Here's how the part is built. I have some questions about the finished solid (model axes, mm). A direction names the side the tool comes from. Give positions to 0.01 mm unless a question says otherwise; leave off trailing zeros. Loops run counter-clockwise (first coordinate to the right, second up) from the corner with the lowest first, then second, coordinate; pieces in that order, holes last. Notation, with made-up numbers: (42.25, -8.75) - (92.25, -8.75) arc R24 ccw to (92.25, 5.25) - close; hole circle Ø2 at (68.5, 71.25). An arc over 180 degrees is marked (long way). Return JSON: item names as keys, results as strings. Group by question number.
(1) For P1, Ø1, axis at y = -360.5, z = 8.5, coming from the -X side; P2, Ø6, axis at y = -316.5, z = 12, coming from the -X side; P3, Ø1.9, axis at y = -411, z = -2, coming from the -X side; P4, Ø8, axis at x = -9, y = -186, coming from the -Z side, each with a flat end and sliding along its axis, tell me the tip position at first contact or that it passes through.
(2) I need wall thicknesses on probe 1 along Y at (x, z) = (-5, 15); probe 2 along Y at (x, z) = (-1.5, 5.75); probe 3 along Z at (x, y) = (0, 1.25). Which ranges of each line are inside material? Lowest first, please. Write a range as [from, to].
(3) If we mould it in two halves opening along Y, with no side actions, what happens to faces 4 (the flat face through (0, -425.018, 6)), 5 (the cylindrical face through (0.385, -300.5, 16.688)), 6 (the flat face through (0, -205.181, 16))? For each: released by +Y, released by -Y, zero draft, split by the parting line, or undercut.
(4) If we section it at B-B (x = -3.5): Please give me the cut outline in (y, z), then the cut area to 3 significant figures.
(5) On a 3-axis mill with a long thin cutter (end or side, diameter ignored), from which of +Z, -Z, +X, -X, +Y, -Y can I reach the whole of each face in a straight line? I mean faces 1 (the cylindrical face through (-0.185, -335.118, 4.438)), 2 (the flat face through (-3, -398.526, 16)), 3 (the cylindrical face through (-0.23, -136.926, 6.495)). Say none if no direction works.
```python
from build123d import *
from build123d import SkipClean  # not in build123d's __all__

# Parameters (mm, degrees)
F1_DEPTH  = 29.21
F3_DEPTH  = 160.5534
F5_DEPTH  = 15.4178
F7_DEPTH  = 42.5196
F9_DEPTH  = 177.3174
F11_DEPTH = 26.4922
F13_DEPTH = 3.1496


with BuildPart() as f1:
    # F0 (on Front) → F1 (new body)
    with BuildSketch(Plane.XZ):
        with BuildLine():
            Line((11.9332703397, -4.6441399077), (17.4498, -4.6441399077))
            Line((17.4498, -4.6441399077), (17.4498, -0.8595399077))
            ThreePointArc((17.4498, -0.8595399077), (0, 16.6918600923), (-17.4498, -0.8595399077))
            Line((-17.4498, -0.8595399077), (-17.4498, -4.6441399077))
            Line((-17.4498, -4.6441399077), (-11.9332703397, -4.6441399077))
            ThreePointArc((-11.9332703397, -4.6441399077), (0, 9.1988600923), (11.9332703397, -4.6441399077))
        make_face()
    extrude(amount=F1_DEPTH)

    # F2 (on face) → F3 (join)
    with BuildSketch(Plane.XZ.offset(29.21)):
        with BuildLine():
            ThreePointArc((-9.1113708093, -4.6441399077), (0, 6.4977884545), (9.1113708093, -4.6441399077))
            Line((9.1113708093, -4.6441399077), (11.9332703397, -4.6441399077))
            ThreePointArc((11.9332703397, -4.6441399077), (0, 9.1988600923), (-11.9332703397, -4.6441399077))
            Line((-11.9332703397, -4.6441399077), (-9.1113708093, -4.6441399077))
        make_face()
        with BuildLine():
            ThreePointArc((-11.9332703397, -4.6441399077), (0, 9.1988600923), (11.9332703397, -4.6441399077))
            Line((11.9332703397, -4.6441399077), (17.4498, -4.6441399077))
            Line((17.4498, -4.6441399077), (17.4498, -0.8595399077))
            ThreePointArc((17.4498, -0.8595399077), (0, 16.6918600923), (-17.4498, -0.8595399077))
            Line((-17.4498, -0.8595399077), (-17.4498, -4.6441399077))
            Line((-17.4498, -4.6441399077), (-11.9332703397, -4.6441399077))
        make_face()
    extrude(amount=F3_DEPTH)

    # F4 (on face) → F5 (join)
    with BuildSketch(Plane.XZ.offset(189.7634)):
        with BuildLine():
            Line((15.9258256822, -4.6441399077), (15.9258256822, -0.850692377))
            ThreePointArc((15.9258256822, -0.850692377), (0, 15.1678600923), (-15.9258256822, -0.850692377))
            Line((-15.9258256822, -0.850692377), (-15.9038025792, -4.6441399077))
            Line((-15.9038025792, -4.6441399077), (-9.1113708093, -4.6441399077))
            ThreePointArc((-9.1113708093, -4.6441399077), (0, 6.4977884545), (9.1113708093, -4.6441399077))
            Line((9.1113708093, -4.6441399077), (15.9258256822, -4.6441399077))
        make_face()
    extrude(amount=F5_DEPTH)

    # F6 (on face) → F7 (join)
    with BuildSketch(Plane.XZ.offset(205.1812)):
        with BuildLine():
            ThreePointArc((-9.1113708093, -4.6441399077), (0, 6.4977884545), (9.1113708093, -4.6441399077))
            Line((9.1113708093, -4.6441399077), (15.9258256822, -4.6441399077))
            Line((15.9258256822, -4.6441399077), (15.9258256822, -0.850692377))
            ThreePointArc((15.9258256822, -0.850692377), (0, 15.1678600923), (-15.9258256822, -0.850692377))
            Line((-15.9258256822, -0.850692377), (-15.9038025792, -4.6441399077))
            Line((-15.9038025792, -4.6441399077), (-9.1113708093, -4.6441399077))
        make_face()
        with BuildLine():
            Line((15.9258256822, -0.850692377), (15.9258256822, -4.6441399077))
            Line((15.9258256822, -4.6441399077), (17.4498, -4.6441399077))
            Line((17.4498, -4.6441399077), (17.4498, -0.8595399077))
            ThreePointArc((17.4498, -0.8595399077), (0, 16.6918600923), (-17.4498, -0.8595399077))
            Line((-17.4498, -0.8595399077), (-17.4498, -4.6441399077))
            Line((-17.4498, -4.6441399077), (-15.9038025792, -4.6441399077))
            Line((-15.9038025792, -4.6441399077), (-15.9258256822, -0.850692377))
            ThreePointArc((-15.9258256822, -0.850692377), (0, 15.1678600923), (15.9258256822, -0.850692377))
        make_face()
    extrude(amount=F7_DEPTH)

    # F8 (on face) → F9 (join)
    with BuildSketch(Plane.XZ.offset(247.7008)):
        with BuildLine():
            ThreePointArc((9.1113708093, -4.6441399077), (0, 6.4977884545), (-9.1113708093, -4.6441399077))
            Line((-9.1113708093, -4.6441399077), (-6.9997961445, -4.6441399077))
            ThreePointArc((-6.9997961445, -4.6441399077), (0, 4.4403884545), (6.9997961445, -4.6441399077))
            Line((6.9997961445, -4.6441399077), (9.1113708093, -4.6441399077))
        make_face()
        with BuildLine():
            ThreePointArc((17.4498, -0.8595399077), (0, 16.6918600923), (-17.4498, -0.8595399077))
            Line((-17.4498, -0.8595399077), (-17.4498, -4.6441399077))
            Line((-17.4498, -4.6441399077), (-9.1113708093, -4.6441399077))
            ThreePointArc((-9.1113708093, -4.6441399077), (0, 6.4977884545), (9.1113708093, -4.6441399077))
            Line((9.1113708093, -4.6441399077), (17.4498, -4.6441399077))
            Line((17.4498, -4.6441399077), (17.4498, -0.8595399077))
        make_face()
    extrude(amount=F9_DEPTH)

    # F10 (on face) → F11 (cut)
    with BuildSketch(Plane.XZ.offset(425.0182)):
        with BuildLine():
            ThreePointArc((0, 15.6758600923), (11.6553662483, 10.8276145233), (16.4338, -0.8565464805))
            Line((16.4338, -0.8565464805), (16.4338, -4.6441399077))
            Line((16.4338, -4.6441399077), (17.4498, -4.6441399077))
            Line((17.4498, -4.6441399077), (17.4498, -0.8595399077))
            ThreePointArc((17.4498, -0.8595399077), (0, 16.6918600923), (-17.4498, -0.8595399077))
            Line((-17.4498, -0.8595399077), (-17.4498, -4.6441399077))
            Line((-17.4498, -4.6441399077), (-16.4338, -4.6441399077))
            Line((-16.4338, -4.6441399077), (-16.4338, -0.8565464804))
            ThreePointArc((-16.4338, -0.8565464804), (-11.6553662483, 10.8276145233), (0, 15.6758600923))
        make_face()
    extrude(amount=-F11_DEPTH, mode=Mode.SUBTRACT)

    # F12 (on face) → F13 (join)
    with BuildSketch(Plane(origin=(0, 0, 0), x_dir=(-1, 0, 0), z_dir=(0, 1, 0))):
        with BuildLine():
            ThreePointArc((16.6878128411, -0.8551161423), (0, 15.9298600923), (-16.6878128411, -0.8551161423))
            Line((-16.6878128411, -0.8551161423), (-16.6878128411, -4.6441399077))
            Line((-16.6878128411, -4.6441399077), (-11.9332703397, -4.6441399077))
            ThreePointArc((-11.9332703397, -4.6441399077), (0, 9.1988600923), (11.9332703397, -4.6441399077))
            Line((11.9332703397, -4.6441399077), (16.6658154206, -4.6441399077))
            Line((16.6658154206, -4.6441399077), (16.6878128411, -0.8551161423))
        make_face()
    with SkipClean():  # cleaning this boolean's faces spoils the solid; the shape is the same uncleaned
        extrude(amount=F13_DEPTH)


solid = f1.part
```
Values:
{
 "1": {"P1": "x = -15.09", "P2": "x = -14.47", "P3": "x = -16.43", "P4": "z = -4.64"},
 "2": {"probe 1": "[-398.53, -205.18], [-189.76, 3.15]", "probe 2": "[-425.02, -247.7]", "probe 3": "[9.2, 15.93]"},
 "3": {"face 4": "released by -Y", "face 5": "zero draft", "face 6": "undercut"},
 "4": {"outline": "(-425.02, 3.54) - (-247.7, 3.54) - (-247.7, 5.81) - (-29.21, 5.81) - (-29.21, 8.68) - (3.15, 8.68) - (3.15, 15.56) - (0, 15.56) - (0, 16.34) - (-189.76, 16.34) - (-189.76, 14.78) - (-205.18, 14.78) - (-205.18, 16.34) - (-398.53, 16.34) - (-398.53, 15.3) - (-425.02, 15.3) - close", "area": "4,760 mm2"},
 "5": {"face 1": "+Y, -Y", "face 2": "+Z, -Y", "face 3": "+Y"}
}
